The figure shows three views and two pictorial views of one solid part (mm, origin at its lowest corner). Answer the questions. A direction names the side the tool comes from. Coordinates: 2 decimals unless noted, no trailing zeros. Order: outer loops, then holes, each group sorted by start corner. A loop starts at its lowest first (then second) coordinate and runs counter-clockwise, first axis right, second up. Notation, with made-up numbers: (88.25, 24.5) - (104.25, 24.5) arc R22 cw to (104.25, 31.5) - close; hole circle Ø5 at (-18.75, -27.5). An arc over 180 degrees is marked (long way). Use one line per item in the form item = value. Start each with the question number.
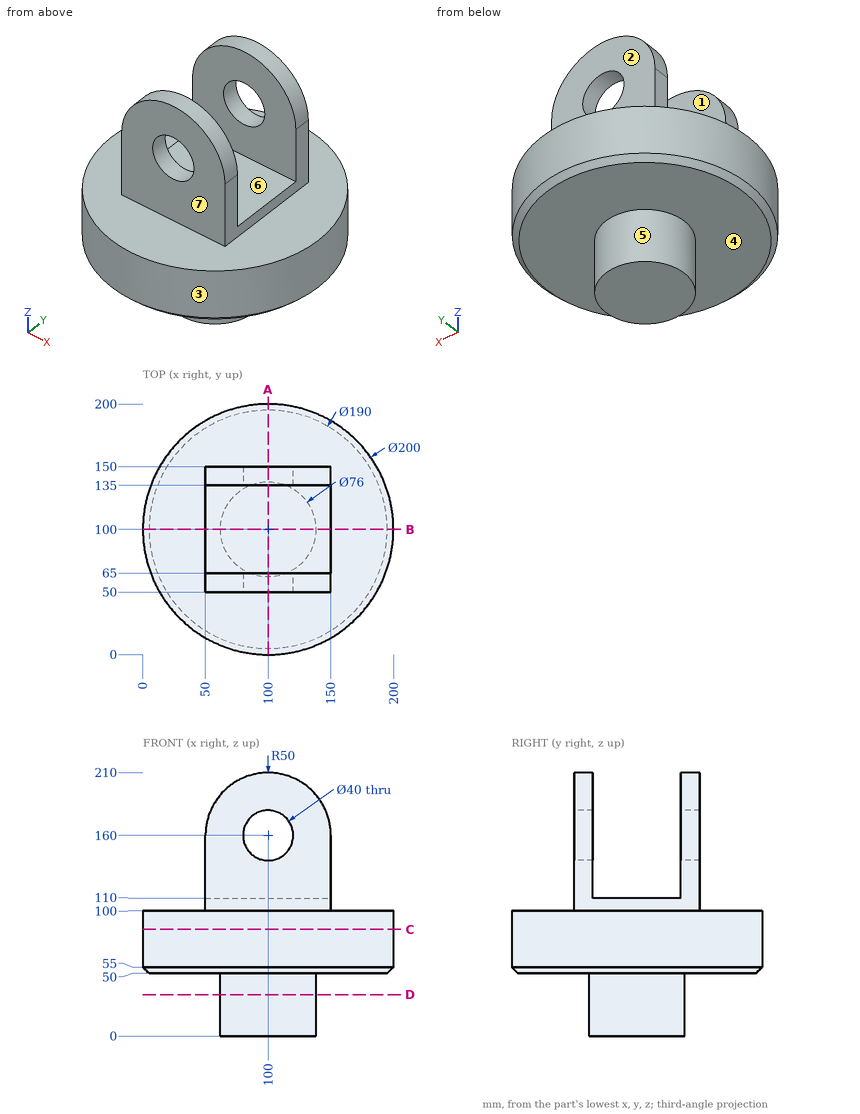
Q1. Given P1, Ø2, axis at x = 109, y = 147, coming from the -Z side; P2, Ø12, axis at x = 49.5, z = 180, coming from the +Y side; P3, Ø10, axis at y = 92, z = 51, coming from the +X side; P4, Ø10, axis at x = 42, z = 145, coming from the +Y side, each flat-ended and moving along its own axis, determine where each tip first touches the part or whether it passes through.
Q2. A cutting plane is placed at D-D (z = 33). Give the vertices of the cut face in (x, y), then the cut area to 3 significant figures.
Q3. Which of the six approach directions +Z, -Z, +X, -X, +Y, -Y give full straight-line access (tool end or side, diameter ignored) to the marked faces 1, 2, 3 and 4?
Q4. Consider probe 1 along Z at (x, y) = (100, 142.5); probe 2 along Y at (x, z) = (141.5, 159.5); probe 3 along Z at (x, y) = (37.5, 112). Determine where each line is inside the solid, lowest interval first.
Q5. For a pull along Y with two mould halves and no side action, classify the marked faces 5, 6 and 7 as +Y half, -Y half, draft (parallel to the pull), parting line (faces both ways), or undercut.
Q6. A cutting plane is placed at B-B (y = 100). Give the vertices of the cut face in (x, z).
Q7. A cutting plane is placed at C-C (z = 85). Give the vertices of the cut face in (x, y), then the cut area to 3 significant figures.
Q8. A cutting plane is placed at A-A (x = 100). Give the vertices of the cut face in (y, z).
Result sheet:
q1.P1 = 50
q1.P2 = 150
q1.P3 = 199.87
q1.P4 = through
q2.outline = circle Ø76 at (100, 100)
q2.area = 4,540 mm^2
q3.face_1 = +Z, +X, -X
q3.face_2 = +Z, +X, -X, +Y
q3.face_3 = +Z, -Z
q3.face_4 = -Z
q4.probe_1 = 50 to 140, 180 to 210
q4.probe_2 = 50 to 65, 135 to 150
q4.probe_3 = 50 to 100
q5.face_5 = parting line
q5.face_6 = undercut
q5.face_7 = -Y half
q6.outline = (0, 55) - (5, 50) - (62, 50) - (62, 0) - (138, 0) - (138, 50) - (195, 50) - (200, 55) - (200, 100) - (150, 100) - (150, 110) - (50, 110) - (50, 100) - (0, 100) - close
q7.outline = circle Ø200 at (100, 100)
q7.area = 31,400 mm^2
q8.outline = (0, 55) - (5, 50) - (62, 50) - (62, 0) - (138, 0) - (138, 50) - (195, 50) - (200, 55) - (200, 100) - (150, 100) - (150, 140) - (135, 140) - (135, 110) - (65, 110) - (65, 140) - (50, 140) - (50, 100) - (0, 100) - close; (50, 180) - (65, 180) - (65, 210) - (50, 210) - close; (135, 180) - (150, 180) - (150, 210) - (135, 210) - close
